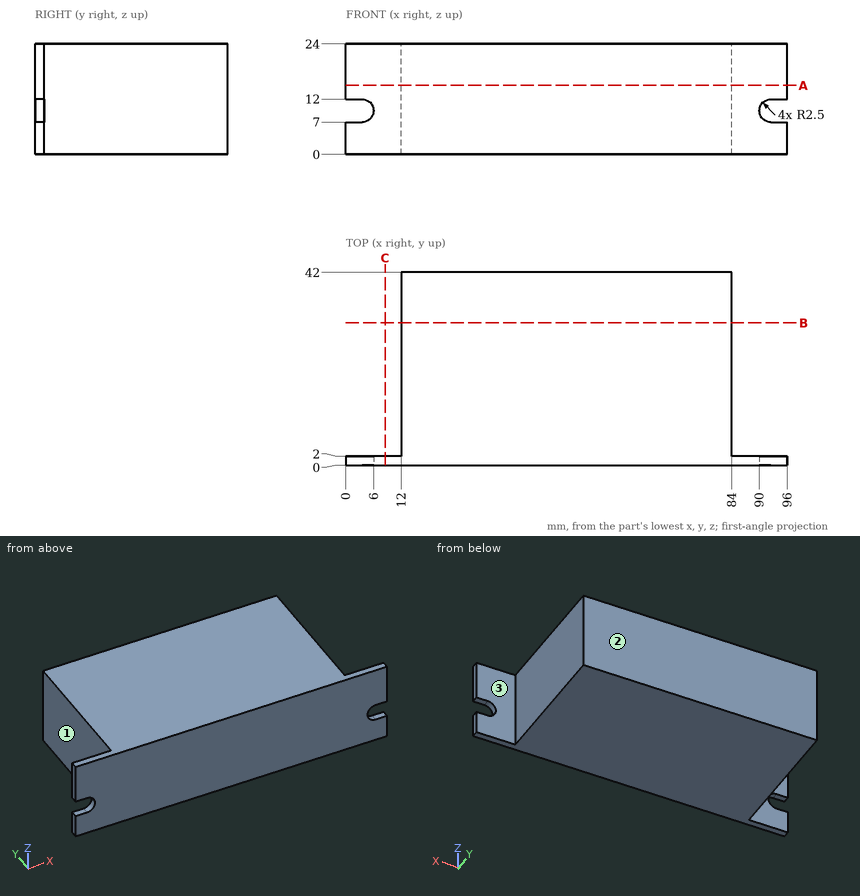
For this review, use the dimensioned drawing (mm, ordinates from the lowest corner) and the shaded views. A direction names the side the tool comes from. Round coordinates to 2 decimals unless told otherwise and drop trailing zeros. Order: outer loops, then holes, each group sorted by start corner. A loop starts at its lowest first (then second) coordinate and runs counter-clockwise, first axis right, second up.
1) Clearance check with flat-ended pins moving along their axes: pin 1 Ø1 at (y, z) = (31.5, 11) entering from +X; pin 2 Ø8 at (y, z) = (9.5, 4) entering from -X. State where each tip first meets the part, or that it passes through.
The answers:
pin 1: stops at x = 84
pin 2: stops at x = 12
2) Consider section B-B (y = 31). State the section outline as (x, z) points, plus the area to 3 significant figures.
The answers:
outline: (12, 0) - (84, 0) - (84, 24) - (12, 24) - close
area: 1,730 mm2
3) For L1, parallel to X at y = 34.5, z = 10; L2, parallel to Y at x = 85, z = 21.5, list the stretches that pass through material, from the lowest coordinate up.
The answers:
L1: x = 12 to 84
L2: y = 0 to 2
4) Consider section A-A (z = 15). State the section outline as (x, y) points.
The answers:
outline: (0, 0) - (96, 0) - (96, 2) - (84, 2) - (84, 42) - (12, 42) - (12, 2) - (0, 2) - close
5) Machinability: for the marked faces 1, 2 and 3, which of the approach directions +Z, -Z, +X, -X, +Y, -Y give a long, thin tool a straight path to every point of the face, cutting with its end or side? Answer none if there is none.
The answers:
face 1: +Z, -Z, -X, +Y
face 2: +Z, -Z, +X, -X, +Y
face 3: +Z, -Z, +X, +Y
6) Consider section C-C (x = 8.5). State the section outline as (y, z) points, plus the area to 3 significant figures.
The answers:
outline: (0, 0) - (2, 0) - (2, 24) - (0, 24) - close
area: 48.0 mm2
